Check sheet for the modelled part. Datum: model origin and axes. Units: mm. A direction names the side the tool comes from. Give positions to 0.01 mm unless a question says otherwise; leave off trailing zeros. Order: outer loops, then holes, each group sorted by start corner. A loop starts at its lowest first (then second) coordinate and runs counter-clockwise, first axis right, second up. Notation, with made-up numbers: M 78.5,65.5 L 96.5,65.5 A24 cw 96.5,83.5 Z; hole C 86.5,-31.75 d11. An arc over 180 degrees is marked long. Return JSON: item names as keys, results as strings. Group by question number.
from build123d import *

# Parameters (mm, degrees)
BOSS_EXTRUDE1_DEPTH = 4
FILLET1_R           = 1


with BuildPart() as part:
    # Sketch1 → Boss-Extrude1 (new body)
    with BuildSketch(Plane(origin=(0, 0, 0), x_dir=(-1, 0, 0), z_dir=(0, 1, 0))):
        Polygon((363.484973911, 0), (0, 0), (-183.030052177, 310), (46.969947823, 310), (138.484973911, 155), (363.484973911, 155), align=None)
        with BuildLine():
            ThreePointArc((288.884973911, 122.1), (290.984973911, 120), (293.084973911, 122.1))
            Line((293.084973911, 122.1), (293.084973911, 147.9))
            ThreePointArc((293.084973911, 147.9), (290.984973911, 150), (288.884973911, 147.9))
            Line((288.884973911, 147.9), (288.884973911, 122.1))
        make_face(mode=Mode.SUBTRACT)
        with BuildLine():
            ThreePointArc((69.152908152, 262.594027053), (69.893566181, 265.470035691), (67.017557543, 266.21069372))
            Line((67.017557543, 266.21069372), (44.800890876, 253.09353998))
            ThreePointArc((44.800890876, 253.09353998), (44.060232847, 250.217531343), (46.936241485, 249.476873314))
            Line((46.936241485, 249.476873314), (69.152908152, 262.594027053))
        make_face(mode=Mode.SUBTRACT)
        with BuildLine():
            ThreePointArc((-110.130052177, 277.1), (-108.030052177, 275), (-105.930052177, 277.1))
            Line((-105.930052177, 277.1), (-105.930052177, 302.9))
            ThreePointArc((-105.930052177, 302.9), (-108.030052177, 305), (-110.130052177, 302.9))
            Line((-110.130052177, 302.9), (-110.130052177, 277.1))
        make_face(mode=Mode.SUBTRACT)
        with BuildLine():
            Line((-25.930052177, 302.9), (-25.930052177, 277.1))
            ThreePointArc((-25.930052177, 277.1), (-28.030052177, 275), (-30.130052177, 277.1))
            Line((-30.130052177, 277.1), (-30.130052177, 302.9))
            ThreePointArc((-30.130052177, 302.9), (-28.030052177, 305), (-25.930052177, 302.9))
        make_face(mode=Mode.SUBTRACT)
        with BuildLine():
            Line((85.474235805, 184.204651092), (107.690902471, 197.321804831))
            ThreePointArc((107.690902471, 197.321804831), (110.566911109, 196.581146802), (109.82625308, 193.705138164))
            Line((109.82625308, 193.705138164), (87.609586413, 180.587984425))
            ThreePointArc((87.609586413, 180.587984425), (84.733577776, 181.328642454), (85.474235805, 184.204651092))
        make_face(mode=Mode.SUBTRACT)
        with BuildLine():
            Line((213.084973911, 147.9), (213.084973911, 122.1))
            ThreePointArc((213.084973911, 122.1), (210.984973911, 120), (208.884973911, 122.1))
            Line((208.884973911, 122.1), (208.884973911, 147.9))
            ThreePointArc((208.884973911, 147.9), (210.984973911, 150), (213.084973911, 147.9))
        make_face(mode=Mode.SUBTRACT)
    extrude(amount=BOSS_EXTRUDE1_DEPTH)

    # Fillet1
    fillet1_edges = [part.edges().sort_by_distance(p)[0] for p in [
        (0, 2, 0),
        (183.030052177, 2, 310),
        (-46.969947823, 2, 310),
        (-138.484973911, 2, 155),
        (-363.484973911, 2, 155),
        (-363.484973911, 2, 0),
    ]]
    fillet(fillet1_edges, radius=FILLET1_R)


solid = part.part
1) Sectioned sample at D-D on z = 30. Record the boundary of the cut face in (x, y), then the cut area to 3 significant figures.
2) Tool access check on faces 1 (the face through (-98.873, 1.972, 187.238)), 2 (the face through (-94, 0, 123)). Record the directions out of +Z, -Z, +X, -X, +Y, -Y that give a thin tool (end or side, any length) a straight path to the whole face; none if there is none.
3) Sectioned sample at A-A on z = 284.5. Record the boundary of the cut face in (x, y).
4) Material ranges on line 1 along X through (y, z) = (0.45, 142); line 2 along X through (y, z) = (3.15, 282); line 3 along Z through (x, y) = (107.5, 0.95), recorded low to high.
5) Sectioned sample at C-C on x = -308.5. Record the boundary of the cut face in (y, z), then the cut area to 3 significant figures.
6) Sectioned sample at B-B on y = 2.9. State how many separate pieces and enclosed holes the cut face has, then the cut area to 3 significant figures.
7) Depth check by flat-ended pin: P1, Ø1, axis at y = 2.5, z = 157, coming from the -X side; P2, Ø2, axis at y = 2.5, z = 293, coming from the -X side; P3, Ø1.5, axis at y = 3, z = 49.5, coming from the +X side. Enter the tip coordinate at first touch or a pass-through.
8) Release check for a two-part mould opening along X. For faces 3 (the face through (-56.06, 1.97, 259.74)), 4 (the face through (89.942, 1.972, 152.336)), 5 (the face through (-92.09, 1.97, 233.58)) record: released by +X, released by -X, zero draft, split by the parting line, or undercut.
Reply:
{
 "1": {"outline": "M -363.48,0 L 17.71,0 L 17.71,4 L -363.48,4 Z", "area": "1,520 mm^2"},
 "2": {"face 1": "+Y, -Y", "face 2": "+Z, -Z, +X, -X, -Y"},
 "3": {"outline": "M -62.03,0 L 25.93,0 L 25.93,4 L -62.03,4 Z; M 30.13,0 L 105.93,0 L 105.93,4 L 30.13,4 Z; M 110.13,0 L 167.97,0 L 167.97,4 L 110.13,4 Z"},
 "4": {"line 1": "-363.48 to -293.08, -288.88 to -213.08, -208.88 to 83.84", "line 2": "-63.5 to 25.93, 30.13 to 105.93, 110.13 to 166.5", "line 3": "182.07 to 275.07, 304.93 to 310"},
 "5": {"outline": "M 0,0 L 4,0 L 4,155 L 0,155 Z", "area": "620 mm^2"},
 "6": {"separate pieces": "1", "enclosed holes": "6", "area": "98,300 mm^2"},
 "7": {"P1": "x = -137.6", "P2": "x = -57.6", "P3": "x = 29.67"},
 "8": {"face 3": "undercut", "face 4": "released by +X", "face 5": "released by -X"}
}
